The drawing under review shows one solid part. Ordinate dimensions are in mm from its lowest x, y, z. A direction names the side the tool comes from. Give positions to 0.01 mm unless a question says otherwise; leave off trailing zeros. Write each loop counter-clockwise with the first axis right and the second up, starting at its lowest first coordinate (ties: lowest second). Pieces come first, ordered by that corner, then holes. Notation, with made-up numbers: M 59,-1 L 84,-1 A26 ccw 84,14 Z; hole C 48.25,-14.5 d9. An arc over 180 degrees is marked long. Write each question's results on one line, items separated by ' | '. Start each with the question number.
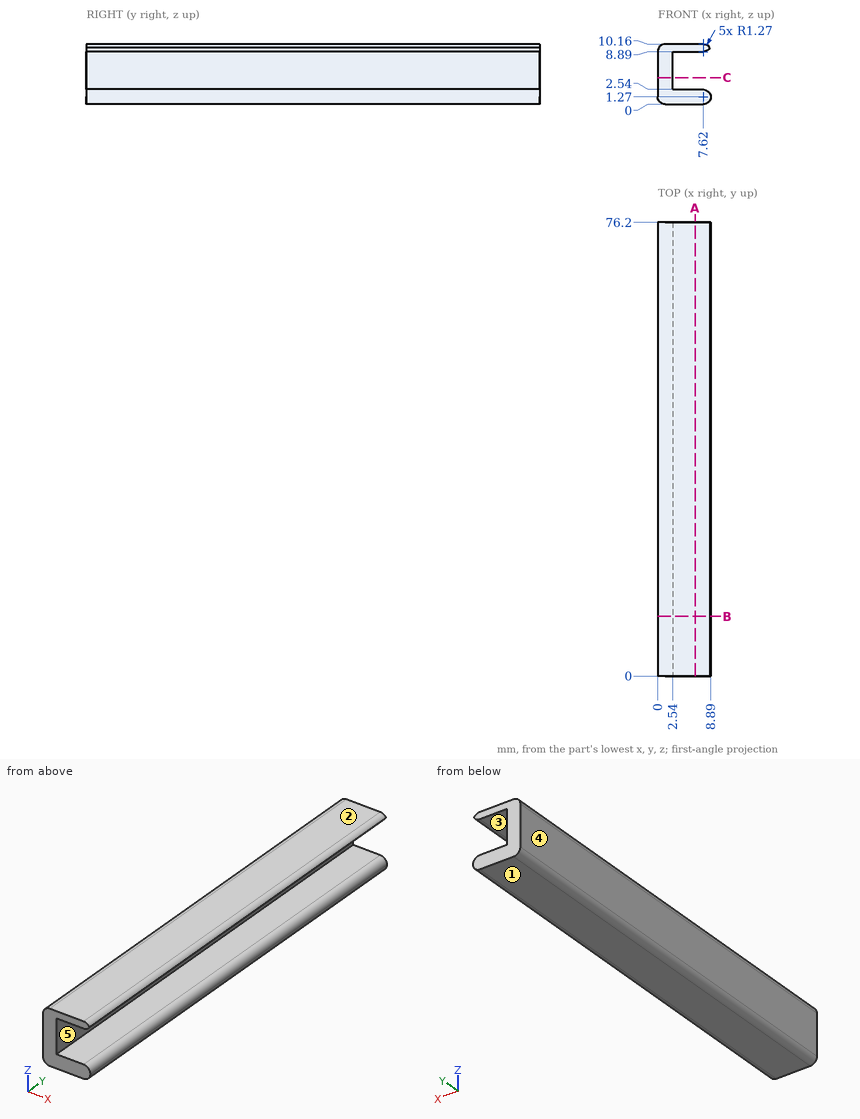
Q1. For pin 1 Ø1.9 at (y, z) = (25.5, 5.5) entering from +X, flat-tipped, find the tip position at first contact; note if it passes through.
Q2. The part is to be moulded in two halves that separate along Z. For the marked faces 1, 2 and 3, say which applies: pulls with the +Z half, pulls with the -Z half, needs draft (parallel to the pull), parting line crosses it, or undercut.
Q3. We need section C-C on z = 4.5. Write out the cut boundary in (x, y).
Q4. We need section B-B on y = 10. Write out the cut boundary in (x, z) (3 decimals), and give its area (3 significant figures).
Q5. For the marked faces 4 and 5, list the 3-axis set-ups (+Z, -Z, +X, -X, +Y, -Y) from which the entire face can be reached by the end or side of a thin tool; tool diameter is ignored.
Q6. We need section A-A on x = 6.25. Write out the cut boundary in (y, z).
Q7. Wall thickness on line 1 along Z through (x, y) = (6.75, 15); line 2 along X through (y, z) = (53, 5.75); line 3 along X through (y, z) = (68.5, 2): over which ranges is each line inside the solid? List them lowest first. Write a range as from..to.
Answer sheet:
1) pin 1: x = 2.54
2) face 1: pulls with the -Z half | face 2: pulls with the +Z half | face 3: undercut
3) outline: M 0,0 L 2.54,0 L 2.54,76.2 L 0,76.2 Z
4) outline: M 0,1.27 A1.27 ccw 1.27,0 L 7.62,0 A1.27 ccw 7.62,2.54 L 2.54,2.54 L 2.54,8.89 L 7.62,8.89 A1.27 ccw 8.72,9.525 A1.27 ccw 7.62,10.16 L 1.27,10.16 A1.27 ccw 0,8.89 Z | area: 48.0 mm^2
5) face 4: +Z, -Z, -X, +Y, -Y | face 5: +X, +Y, -Y
6) outline: M 0,0 L 76.2,0 L 76.2,2.54 L 0,2.54 Z; M 0,8.89 L 76.2,8.89 L 76.2,10.16 L 0,10.16 Z
7) line 1: 0..2.54, 8.89..10.16 | line 2: 0..2.54 | line 3: 0..8.66
